Geometry: see drawing. Coordinates: mm, zero at the bounding-box minimum. Round coordinates to 2 decimals unless told otherwise and drop trailing zeros. Order: outer loops, then holes, each group sorted by start corner. A loop starts at its lowest first (then second) coordinate and runs counter-clockwise, first axis right, second up. Notation, with made-up numbers: (-19.5, -29) - (-8.5, -29) arc R16 cw to (-8.5, -18) - close; hole circle Ø6 at (-17.5, 55.5). An arc over 180 degrees is marked (long way). Put each result on its own line as item: value. Start each with the question number.
1) Section A-A on y = 66. Output: boundary loops of the cut face in (x, z), then the cut area to 3 significant figures.
2) Contact query for a flat-ended pin moving along its axis: P1, Ø5, axis at x = 1477, y = 196.5, coming from the -Z side. Output: stop coordinate, or through.
3) Line query: probe 1 along Z at (x, y) = (445, 85); probe 2 along X at (y, z) = (264, 455.5). Output: solid intervals per line, ascending. Write a range as [from, to].
4) Mould query, pull axis X, two halves, no side actions, for the marked faces 1 and 2. Classes: +X half, -X half, draft (parallel to the pull), parting line (faces both ways), or undercut.
5) Section C-C on x = 676.5. Output: boundary loops of the cut face in (y, z), then the cut area to 3 significant figures.
6) Section B-B on z = 440.5. Output: boundary loops of the cut face in (x, y), then the cut area to 3 significant figures.
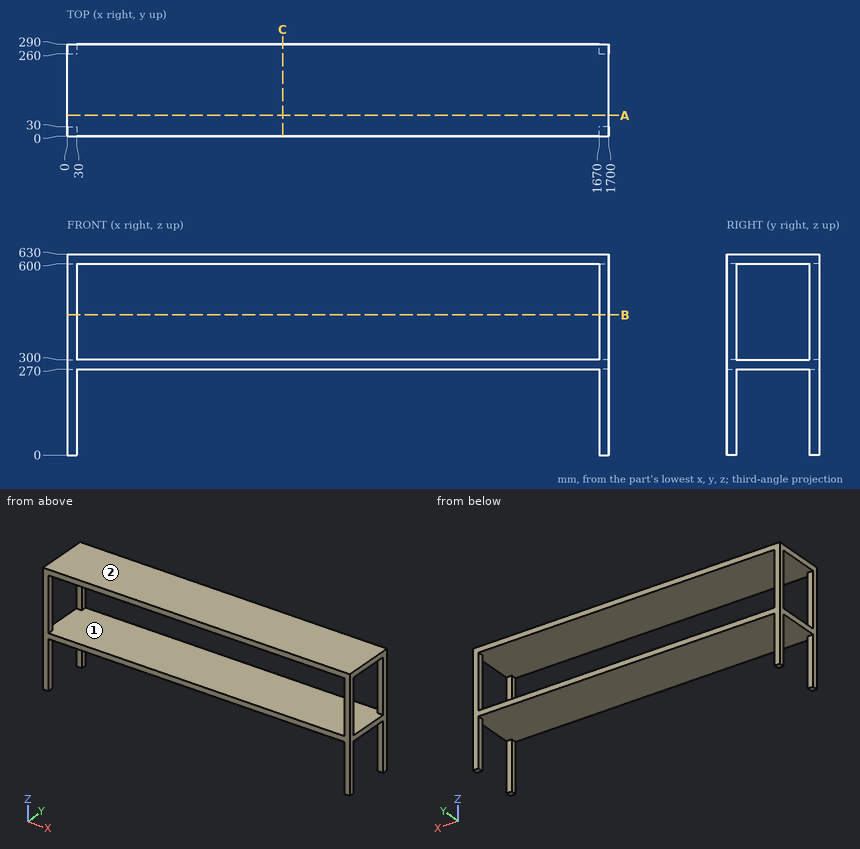
Answer sheet:
1. outline: (0, 270) - (1700, 270) - (1700, 300) - (0, 300) - close; (0, 600) - (1700, 600) - (1700, 630) - (0, 630) - close
1. area: 102,000 mm^2
2. P1: z = 270
3. probe 1: [270, 300], [600, 630]
3. probe 2: [0, 30], [1670, 1700]
4. face 1: undercut
4. face 2: draft
5. outline: (0, 270) - (290, 270) - (290, 300) - (0, 300) - close; (0, 600) - (290, 600) - (290, 630) - (0, 630) - close
5. area: 17,400 mm^2
6. outline: (0, 0) - (30, 0) - (30, 30) - (0, 30) - close; (0, 260) - (30, 260) - (30, 290) - (0, 290) - close; (1670, 0) - (1700, 0) - (1700, 30) - (1670, 30) - close; (1670, 260) - (1700, 260) - (1700, 290) - (1670, 290) - close
6. area: 3,600 mm^2
